Design review of the part built by this model. Coordinates are the model's own, in mm. A direction names the side the tool comes from. Give positions to 0.01 mm unless a question says otherwise; leave off trailing zeros. Loops run counter-clockwise (first coordinate to the right, second up) from the corner with the lowest first, then second, coordinate; pieces in that order, holes last. Notation, with made-up numbers: (32.5, -25) - (89.5, -25) arc R19 cw to (89.5, 5) - close; hole circle Ø1 at (-22, 59). An arc over 180 degrees is marked (long way). One line per item, written item: value. Start each with the question number.
```python
from build123d import *

# Parameters (mm, degrees)
F0_R     = 1.7
F0_R_2   = 1.5
F1_DEPTH = 54.45
F2_R     = 1.7
F3_DEPTH = 44
F4_R     = 1.7
F5_DEPTH = 44
F6_R     = 5
F7_DEPTH = 55
F8_DEPTH = 5


with BuildPart() as f1:
    # F0 (on Top) → F1 (new body)
    with BuildSketch(Plane.XY):
        with BuildLine():
            Line((18, 22), (-22, 22))
            Line((-22, 22), (-22, -22))
            Line((-22, -22), (22, -22))
            Line((22, -22), (22, 18))
            ThreePointArc((22, 18), (15.171573, 15.171573), (18, 22))
        make_face()
        with Locations((-17, -10)):
            Circle(F0_R, mode=Mode.SUBTRACT)
        with Locations((0, -16)):
            Circle(F0_R_2, mode=Mode.SUBTRACT)
        with Locations((3, -10)):
            Circle(F0_R, mode=Mode.SUBTRACT)
        with Locations((-17, -10)):
            Circle(F0_R)
        with Locations((0, -16)):
            Circle(F0_R_2)
        with Locations((3, -10)):
            Circle(F0_R)
    extrude(amount=-F1_DEPTH)

    # F2 (on face) → F3 (cut)
    with BuildSketch(Plane.XZ.offset(22)):
        with Locations((-12, -25)):
            Circle(F2_R)
        with Locations((12, -25)):
            Circle(F2_R)
    extrude(amount=-F3_DEPTH, mode=Mode.SUBTRACT)

    # F4 (on face) → F5 (cut)
    with BuildSketch(Plane.YZ.offset(22)):
        with Locations((-12, -12)):
            Circle(F4_R)
        with Locations((12, -12)):
            Circle(F4_R)
    extrude(amount=-F5_DEPTH, mode=Mode.SUBTRACT)

    # F6
    f6_edges = [f1.edges().sort_by_distance(p)[0] for p in [
        (22, -22, -27.225),
        (-22, -22, -27.225),
        (-22, 22, -27.225),
    ]]
    fillet(f6_edges, radius=F6_R)

    # F0 (on Top) → F7 (cut)
    with BuildSketch(Plane.XY):
        with Locations((0, -16)):
            Circle(F0_R_2)
    extrude(amount=-F7_DEPTH, mode=Mode.SUBTRACT)

    # F0 (on Top) → F8 (cut)
    with BuildSketch(Plane.XY):
        with Locations((-17, -10)):
            Circle(F0_R)
        with Locations((3, -10)):
            Circle(F0_R)
    extrude(amount=-F8_DEPTH, mode=Mode.SUBTRACT)


solid = f1.part
```
(1) Take a section at A-A on x = 0. State the section outline as (y, z) points.
(2) For pin 1 Ø5.5 at (x, z) = (12, -25) entering from +Y; pin 2 Ø3 at (y, z) = (-12, -12) entering from +X; pin 3 Ø2 at (x, y) = (3, -10) entering from +Z, all flat-tipped, find the tip position at first contact; note any pin that passes through.
(3) Take a section at C-C on z = -45. State the section outline as (x, y) points.
(4) Machinability: for faces 1 (the flat face through (-17, -10, -5)), 2 (the cylindrical face through (0.31, -10.43, -12.65)), which of the approach directions +Z, -Z, +X, -X, +Y, -Y give a long, thin tool a straight path to every point of the face, cutting with its end or side? Answer none if there is none.
(5) To check wall thickness, follow L1, parallel to Z at x = -12, y = 15; L2, parallel to Y at x = 0, z = -32; L3, parallel to Z at x = 1, y = -12. State the ranges of each line that lie inside material, in increasing order. Write a range as from..to.
(6) Draft analysis for pull direction Y (two halves, no side actions). For faces 3 (the cylindrical face through (21, -20, -28)), 4 (the cylindrical face through (15.266, 15.08, -26.844)), 5 (the flat face through (22, 0, -27)), state which applies: pulls with the +Y half, pulls with the -Y half, needs draft (parallel to the pull), parting line crosses it, or undercut.
(7) Take a section at B-B on y = -16. State the section outline as (x, z) points.
Here are the results:
1. outline: (-22, -54.45) - (-17.5, -54.45) - (-17.5, 0) - (-22, 0) - close; (-14.5, -54.45) - (22, -54.45) - (22, 0) - (-14.5, 0) - close; hole circle Ø3.4 at (-12, -12); hole circle Ø3.4 at (12, -12)
2. pin 1: y = 22
2. pin 2: through
2. pin 3: z = -5
3. outline: (-22, -17) arc R5 ccw to (-17, -22) - (17, -22) arc R5 ccw to (22, -17) - (22, 18) arc R4 cw (long way) to (18, 22) - (-17, 22) arc R5 ccw to (-22, 17) - close; hole circle Ø3 at (0, -16)
4. face 1: +Z
4. face 2: +X, -X
5. L1: -54.45..-26.7, -23.3..0
5. L2: -22..-17.5, -14.5..22
5. L3: -54.45..-13.7, -10.3..0
6. face 3: pulls with the -Y half
6. face 4: undercut
6. face 5: needs draft
7. outline: (-22, -54.45) - (-1.5, -54.45) - (-1.5, 0) - (-22, 0) - close; (1.5, -54.45) - (22, -54.45) - (22, 0) - (1.5, 0) - close; hole circle Ø3.4 at (-12, -25); hole circle Ø3.4 at (12, -25)
